Design review of the part built by this model. Coordinates are the model's own, in mm. Face numbers are marked on the shaded views. Give positions to 0.01 mm unless a question says otherwise; leave off trailing zeros. Write each loop counter-clockwise with the first axis right and the second up, starting at its lowest first coordinate (ties: lowest second). Pieces come first, ordered by that corner, then holes. Notation, with made-up numbers: M -23,-6.5 L 29,-6.5 A19 ccw 29,8.5 Z; hole C -20.75,44 d1. An arc over 180 degrees is marked long. One line per item, written item: value. Start each with the question number.
```python
from build123d import *

# Parameters (mm, degrees)
F0_R     = 18.1702284577
F1_DEPTH = 6.5465988591
F2_R     = 4
F3_R     = 2
F4_T     = -1


# Not quite as in the source:
# - a shell that OpenCascade refuses in one call is made with other operations: the cavity is built on its own and cut out


with BuildPart() as f1:
    # F0 (on Top) → F1 (new body)
    with BuildSketch(Plane.XY):
        Circle(F0_R)
    extrude(amount=F1_DEPTH)

    # F2
    f2_edges = [f1.edges().sort_by_distance(p)[0] for p in [
        (-18.170228, 0, 0),
    ]]
    fillet(f2_edges, radius=F2_R)

    # F3
    f3_edges = [f1.edges().sort_by_distance(p)[0] for p in [
        (-18.170228, 0, 6.546599),
    ]]
    fillet(f3_edges, radius=F3_R)

    # F4: a shell. OpenCascade refuses it in one call, so the cavity is built on its own and cut out:
    # the body offset inwards by the wall thickness, plus a prism from it out through each open face.
    f4_core = offset(f1.part, amount=F4_T, mode=Mode.PRIVATE)
    f4_exits = [f4_core.faces().sort_by_distance(p)[0] for p in [
        (0, 0, 5.546599),
    ]]
    add(f4_core, mode=Mode.SUBTRACT)
    extrude(f4_exits, amount=-F4_T, mode=Mode.SUBTRACT)


solid = f1.part
```
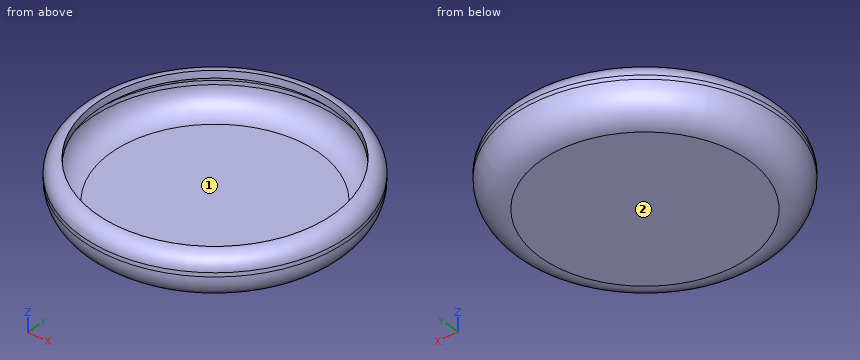
Q1. The part is to be moulded in two halves that separate along Y. For the marked faces 1 and 2, say which applies: pulls with the +Y half, pulls with the -Y half, needs draft (parallel to the pull), parting line crosses it, or undercut.
Q2. Wall thickness on line 1 (Y direction, x = 0, z = 4.45); line 2 (Z direction, x = 8, y = 0.5); line 3 (Y direction, x = -6, z = 4.5): over which ranges is each line inside the solid? List them lowest first. Write a range as from..to.
Q3. Take a section at D-D, the plane z = 2. Give the boundary of the cut face in (x, y), then the cut area to 3 significant figures.
Q4. For P1, Ø1, axis at x = -2, y = -11.5, coming from the +Z side; P2, Ø2, axis at x = -5, z = 2.5, coming from the -Y side; P3, Ø2, axis at y = 3, z = 4.5, coming from the -X side, all flat-tipped, find the tip position at first contact; note any pin that passes through.
Q5. Take a section at C-C, the plane z = 5. Give the boundary of the cut face in (x, y), then the cut area to 3 significant figures.
Q6. Take a section at A-A, the plane x = 0. Give the boundary of the cut face in (y, z).
Results list:
1. face 1: undercut
1. face 2: needs draft
2. line 1: y = -18.17..-17.17, 17.17..18.17
2. line 2: z = 0..1
2. line 3: y = -17.15..-16.09, 16.09..17.15
3. outline: C 0,0 d35.27; hole C 0,0 d32.81
3. area: 131 mm^2
4. P1: stops at z = 1
4. P2: stops at y = -17.57
4. P3: stops at x = -18.06
5. outline: C 0,0 d36.24; hole C 0,0 d34.12
5. area: 117 mm^2
6. outline: M -18.17,4 A4 ccw -14.17,0 L 14.17,0 A4 ccw 18.17,4 L 18.17,4.55 A2 ccw 16.17,6.55 L 16.17,5.55 A1 cw 17.17,4.55 L 17.17,4 A3 cw 14.17,1 L -14.17,1 A3 cw -17.17,4 L -17.17,4.55 A1 cw -16.17,5.55 L -16.17,6.55 A2 ccw -18.17,4.55 Z
